Work out the finished part from the listing and answer in its coordinate system (mm). A direction names the side the tool comes from. Round coordinates to 2 decimals unless told otherwise and drop trailing zeros. Order: outer loops, then holes, each group sorted by start corner. A loop starts at its lowest first (then second) coordinate and runs counter-clockwise, first axis right, second up. Notation, with made-up numbers: (-1.5, 43.5) - (53.5, 43.5) arc R6 ccw to (53.5, 49.5) - close; hole circle Ø7 at (-36, 86.25). An arc over 180 degrees is marked (long way). Use one line per item in the form item = value. Start each with the question number.
Q1. Which of the six approach directions +Z, -Z, +X, -X, +Y, -Y give full straight-line access (tool end or side, diameter ignored) to faces 4 (the flat face through (-19, 9, -34)), 5 (the flat face through (-42, 15, -2)), 6 (the flat face through (44, 16, 0)), 7 (the flat face through (-29, 24, 34))?
Q2. The part is cut by section B-B on x = 8.5. Determine the outline of the cut face in (y, z), plus the area to 3 significant figures.
Q3. For a pull along Y with two mould halves and no side action, classify faces 1 (the flat face through (-1, 30, 0)), 2 (the flat face through (-14, 17, -34)), 3 (the flat face through (5, 15, -33)) as +Y half, -Y half, draft (parallel to the pull), parting line (faces both ways), or undercut.
Q4. The part is cut by section A-A on y = 20. Determine the outline of the cut face in (x, z), plus the area to 3 significant figures.
Q5. The part is cut by section D-D on y = 10.5. Determine the outline of the cut face in (x, z), plus the area to 3 significant figures.
Q6. The part is cut by section C-C on z = -19. Determine the outline of the cut face in (x, y).
Q7. Find the intervals of material crossed by line 1 (X direction, y = 3, z = -12); line 2 (Z direction, x = 7.5, y = 9); line 3 (X direction, y = 2, z = -31), in increasing order. Write a range as [from, to].
Q8. Given P1, Ø2, axis at x = 12.5, z = 23, coming from the -Y side; P2, Ø1.2, axis at x = -31.5, z = -31, coming from the -Y side; P3, Ø1.5, axis at x = -18, y = 14, coming from the -Z side, each flat-ended and moving along its own axis, determine where each tip first touches the part or whether it passes through.
from build123d import *

# Parameters (mm, degrees)
SKETCH1_W                 = 88
SKETCH1_H                 = 70
BOSS_EXTRUDE1_DEPTH       = 32
SKETCH2_W                 = 84
SKETCH2_H                 = 66
CUT_EXTRUDE1_DEPTH        = 30
SKETCH4_W                 = 10
SKETCH4_H                 = 16.5
CUT_EXTRUDE2_DEPTH        = 3
SKETCH6_W                 = 10
SKETCH6_H                 = 10
CUT_EXTRUDE3_DEPTH        = 3
SKETCH7_W                 = 86
SKETCH7_H                 = 68
CUT_EXTRUDE4_DEPTH        = 1
SKETCH10_W                = 25
SKETCH10_H                = 6.5
SKETCH10_W_2              = 6
SKETCH10_H_2              = 6
CUT_EXTRUDE5_DEPTH        = 3
BOSS_EXTRUDE2_DEPTH       = 30
F_2_0MM_DOWEL_HOLE1_D     = 1.5
F_2_0MM_DOWEL_HOLE1_DEPTH = 2.749354536
F_2_0MM_DOWEL_HOLE1_TIP   = 0.450645464
CUT_EXTRUDE6_DEPTH        = 3


with BuildPart() as part:
    # Sketch1 → Boss-Extrude1 (new body)
    with BuildSketch(Plane(origin=(0, 0, 0), x_dir=(1, 0, 0), z_dir=(0, 1, 0))):
        Rectangle(SKETCH1_W, SKETCH1_H)
    extrude(amount=BOSS_EXTRUDE1_DEPTH)

    # Sketch2 → Cut-Extrude1 (cut)
    with BuildSketch(Plane(origin=(0, 0, 0), x_dir=(1, 0, 0), z_dir=(0, 1, 0))):
        Rectangle(SKETCH2_W, SKETCH2_H)
    extrude(amount=CUT_EXTRUDE1_DEPTH, mode=Mode.SUBTRACT)

    # Sketch4 → Cut-Extrude2 (cut)
    with BuildSketch(Plane(origin=(0, 0, -35), x_dir=(-1, 0, 0), z_dir=(0, 0, -1))):
        with Locations((19, 17.25)):
            Rectangle(SKETCH4_W, SKETCH4_H)
    extrude(amount=-CUT_EXTRUDE2_DEPTH, mode=Mode.SUBTRACT)

    # Sketch6 → Cut-Extrude3 (cut)
    with BuildSketch(Plane.XY.offset(35)):
        with Locations((-29, 19)):
            Rectangle(SKETCH6_W, SKETCH6_H)
    extrude(amount=-CUT_EXTRUDE3_DEPTH, mode=Mode.SUBTRACT)

    # Sketch7 → Cut-Extrude4 (cut)
    with BuildSketch(Plane.XZ):
        Rectangle(SKETCH7_W, SKETCH7_H)
    extrude(amount=-CUT_EXTRUDE4_DEPTH, mode=Mode.SUBTRACT)

    # Sketch10 → Cut-Extrude5 (cut)
    with BuildSketch(Plane(origin=(0, 0, -35), x_dir=(-1, 0, 0), z_dir=(0, 0, -1))):
        with Locations((-26.5, 25.25)):
            Rectangle(SKETCH10_W, SKETCH10_H)
        with Locations((-13, 4.5)):
            Rectangle(SKETCH10_W_2, SKETCH10_H_2)
    extrude(amount=-CUT_EXTRUDE5_DEPTH, mode=Mode.SUBTRACT)

    # Sketch11 → Boss-Extrude2 (add)
    with BuildSketch(Plane.XZ.offset(-30)):
        with BuildLine():
            Line((38, 33), (42, 33))
            Line((42, 33), (42, 29))
            ThreePointArc((42, 29), (39.171572875, 30.171572875), (38, 33))
        make_face()
        with BuildLine():
            Line((-42, 33), (-42, 29))
            ThreePointArc((-42, 29), (-39.171572875, 30.171572875), (-38, 33))
            Line((-38, 33), (-42, 33))
        make_face()
        with BuildLine():
            Line((42, -29.5), (42, -33))
            Line((42, -33), (38.5, -33))
            ThreePointArc((38.5, -33), (39.525126266, -30.525126266), (42, -29.5))
        make_face()
        with BuildLine():
            Line((-35.5, -33), (-27.5, -33))
            ThreePointArc((-27.5, -33), (-31.5, -29), (-35.5, -33))
        make_face()
    extrude(amount=BOSS_EXTRUDE2_DEPTH)

    # Ø2.0mm Dowel Hole1
    with Locations(Plane(origin=(0, 0, 0), x_dir=(-1, 0, 0), z_dir=(0, -1, 0))):
        with Locations((-41, 31), (31.5, 31), (40.267949192, -32), (-40, -32)):
            Hole(F_2_0MM_DOWEL_HOLE1_D / 2, depth=F_2_0MM_DOWEL_HOLE1_DEPTH)
            with Locations((0, 0, -(F_2_0MM_DOWEL_HOLE1_DEPTH + F_2_0MM_DOWEL_HOLE1_TIP / 2))):  # 118° drill point
                Cone(0, F_2_0MM_DOWEL_HOLE1_D / 2, F_2_0MM_DOWEL_HOLE1_TIP, mode=Mode.SUBTRACT)

    # Sketch22 → Cut-Extrude6 (cut)
    with BuildSketch(Plane(origin=(0, 0, -35), x_dir=(-1, 0, 0), z_dir=(0, 0, -1))):
        with BuildLine():
            Line((37.9, 24.08), (37.9, 18.3))
            ThreePointArc((37.9, 18.3), (39.18, 17.02), (40.46, 18.3))
            Line((40.46, 18.3), (40.46, 24.08))
            ThreePointArc((40.46, 24.08), (39.18, 25.36), (37.9, 24.08))
        make_face()
    extrude(amount=-CUT_EXTRUDE6_DEPTH, mode=Mode.SUBTRACT)


solid = part.part
Found:
q1.face_4 = -Z
q1.face_5 = -Y
q1.face_6 = +Z, -Z, +X, +Y, -Y
q1.face_7 = +Z
q2.outline = (0, -35) - (32, -35) - (32, 35) - (0, 35) - (0, 34) - (1, 34) - (1, 33) - (30, 33) - (30, -33) - (1, -33) - (1, -34) - (0, -34) - close
q2.area = 258 mm²
q3.face_1 = -Y half
q3.face_2 = undercut
q3.face_3 = draft
q4.outline = (-44, -35) - (-40.46, -35) - (-40.46, -33) - (-42, -33) - (-42, 29) arc R4 ccw to (-38, 33) - (-34, 33) - (-34, 35) - (-44, 35) - close; (-37.9, -35) - (-24, -35) - (-24, -33) - (-27.5, -33) arc R4 ccw to (-35.5, -33) - (-37.9, -33) - close; (-24, 33) - (38, 33) arc R4 ccw to (42, 29) - (42, -29.5) arc R3.5 ccw to (38.5, -33) - (-14, -33) - (-14, -35) - (44, -35) - (44, 35) - (-24, 35) - close
q4.area = 631 mm²
q5.outline = (-44, -35) - (-24, -35) - (-24, -33) - (-27.5, -33) arc R4 ccw to (-35.5, -33) - (-42, -33) - (-42, 29) arc R4 ccw to (-38, 33) - (38, 33) arc R4 ccw to (42, 29) - (42, -29.5) arc R3.5 ccw to (38.5, -33) - (-14, -33) - (-14, -35) - (44, -35) - (44, 35) - (-44, 35) - close
q5.area = 656 mm²
q6.outline = (-44, 0) - (-43, 0) - (-43, 1) - (-42, 1) - (-42, 30) - (42, 30) - (42, 1) - (43, 1) - (43, 0) - (44, 0) - (44, 32) - (-44, 32) - close
q7.line_1 = [-44, -42], [42, 44]
q7.line_2 = [-35, -33], [33, 35]
q7.line_3 = [-44, -42], [-34.96, -32.25], [-30.75, -28.04], [39.13, 40.25], [41.75, 44]
q8.P1 = 30
q8.P2 = 2.84
q8.P3 = 33
